Design review of the part built by this model. Coordinates are the model's own, in mm. A direction names the side the tool comes from. Give positions to 0.01 mm unless a question says otherwise; leave off trailing zeros. Write each loop counter-clockwise with the first axis right and the second up, starting at its lowest first coordinate (ties: lowest second). Pieces come first, ordered by that corner, then holes.
```python
from build123d import *

# Parameters (mm, degrees)
SCHIZZO1_R                   = 15
ESTRUSIONE_ESTRUSIONE1_DEPTH = 3.781092502
SCHIZZO2_R                   = 1.625
SCHIZZO2_R_2                 = 1.3
TAGLIO_ESTRUSIONE1_DEPTH     = 4.781092502
SCHIZZO3_R                   = 1.3
TAGLIO_ESTRUSIONE2_DEPTH     = 1.6


with BuildPart() as part:
    # Schizzo1 → Estrusione-Estrusione1 (new body)
    with BuildSketch(Plane.XY):
        Circle(SCHIZZO1_R)
    extrude(amount=ESTRUSIONE_ESTRUSIONE1_DEPTH)

    # Schizzo2 → Taglio-Estrusione1 (cut, through all)
    with BuildSketch(Plane.XY.offset(3.781092502)):
        with Locations((12, 0)):
            Circle(SCHIZZO2_R)
        with Locations((-6, 10.392304845)):
            Circle(SCHIZZO2_R)
        with Locations((-6, -10.392304845)):
            Circle(SCHIZZO2_R)
        Circle(SCHIZZO2_R_2)
    extrude(amount=-TAGLIO_ESTRUSIONE1_DEPTH, mode=Mode.SUBTRACT)

    # Schizzo3 → Taglio-Estrusione2 (cut)
    with BuildSketch(Plane.XY.offset(3.781092502)):
        with BuildLine():
            Line((2.324693054, 3.969357908), (-7.234922947, -1.579015265))
            ThreePointArc((-7.234922947, -1.579015265), (-8.052751546, -4.652222254), (-4.980479907, -5.473557626))
            Line((-4.980479907, -5.473557626), (7.230479097, 1.576442841))
            ThreePointArc((7.230479097, 1.576442841), (8.058653282, 4.641964906), (4.996568233, 5.482758079))
            Line((4.996568233, 5.482758079), (2.324693054, 3.969357908))
        make_face()
        Circle(SCHIZZO3_R, mode=Mode.SUBTRACT)
        with BuildLine():
            Line((-4.599733028, -0.049558742), (-1.133047311, 1.962495511))
            Line((-1.133047311, 1.962495511), (-2.3, 3.983716857))
            ThreePointArc((-2.3, 3.983716857), (-3.996048921, 2.278506752), (-4.599733028, -0.049558742))
        make_face()
        with BuildLine():
            Line((-2.3, 3.983716857), (-1.133047311, 1.962495511))
            Line((-1.133047311, 1.962495511), (2.324693054, 3.969357908))
            ThreePointArc((2.324693054, 3.969357908), (0.014282212, 4.599977828), (-2.3, 3.983716857))
        make_face()
        with BuildLine():
            ThreePointArc((-2.349640269, -3.954641653), (2.3, -3.983716857), (4.599640269, 0.057527336))
            Line((4.599640269, 0.057527336), (-2.349640269, -3.954641653))
        make_face()
    extrude(amount=-TAGLIO_ESTRUSIONE2_DEPTH, mode=Mode.SUBTRACT)


solid = part.part
```
(1) Mouldability with a two-part tool opening along Y and no side actions: class faces 3 (the face through (3, 0, 0)), 4 (the face through (-14.985, 0.66, 1.864)), 5 (the face through (-0.17, 1.29, 1.11)), 6 (the face through (10.377, 0.071, 1.917)) as pulls with the +Y half, pulls with the -Y half, needs draft (parallel to the pull), parting line crosses it, or undercut.
Resolved:
face 3: needs draft
face 4: parting line crosses it
face 5: undercut
face 6: undercut
(2) Clearance check with flat-ended pins moving along their axes: P1, Ø1.6, axis at x = 0, y = 0, coming from the -Z side; P2, Ø1, axis at y = -4, z = 0.5, coming from the +X side; P3, Ø1, axis at x = 6, z = 2, coming from the -Y side; P4, Ø2, axis at x = 4.5, z = 2.5, coming from the +Y side. State where each tip first meets the part, or that it passes through.
Resolved:
P1: passes through
P2: stops at x = 14.59
P3: stops at y = -13.96
P4: stops at y = 14.59
(3) Consider section D-D, the plane z = 2.9. Give the boundary of the cut face in (x, y) (3 decimals), then the cut area to 3 significant figures.
Resolved:
outline: circle Ø30 at (0, 0); hole circle Ø3.25 at (-6, -10.392); hole circle Ø3.25 at (-6, 10.392); hole (-7.235, -1.579) arc R2.25 ccw to (-4.98, -5.474) - (-2.35, -3.955) arc R4.6 ccw to (4.6, 0.058) - (7.23, 1.576) arc R2.25 ccw to (4.997, 5.483) - (2.325, 3.969) arc R4.6 ccw to (-4.6, -0.05) - close; hole circle Ø3.25 at (12, 0)
area: 576 mm2
(4) Consider section B-B, the plane x = -6. Give the boundary of the cut face in (y, z), then the cut area to 3 significant figures.
Resolved:
outline: (-13.75, 0) - (-12.02, 0) - (-12.02, 3.78) - (-13.75, 3.78) - close; (-8.77, 0) - (8.77, 0) - (8.77, 3.78) - (-0.86, 3.78) - (-0.86, 2.18) - (-5.77, 2.18) - (-5.77, 3.78) - (-8.77, 3.78) - close; (12.02, 0) - (13.75, 0) - (13.75, 3.78) - (12.02, 3.78) - close
area: 71.5 mm2
(5) Consider section C-C, the plane y = 0.75. Give the boundary of the cut face in (x, z).
Resolved:
outline: (-14.98, 0) - (-1.06, 0) - (-1.06, 2.18) - (-4.54, 2.18) - (-4.54, 3.78) - (-14.98, 3.78) - close; (1.06, 0) - (10.56, 0) - (10.56, 3.78) - (5.8, 3.78) - (5.8, 2.18) - (1.06, 2.18) - close; (13.44, 0) - (14.98, 0) - (14.98, 3.78) - (13.44, 3.78) - close
(6) To check wall thickness, follow L1, parallel to Y at x = 0, z = 1.6; L2, parallel to Y at x = -6, z = 2.9; L3, parallel to Y at x = -6, z = 2.05. State the ranges of each line that lie inside material, in increasing order.
Resolved:
L1: y = -15 to -1.3, 1.3 to 15
L2: y = -13.75 to -12.02, -8.77 to -5.77, -0.86 to 8.77, 12.02 to 13.75
L3: y = -13.75 to -12.02, -8.77 to 8.77, 12.02 to 13.75
(7) Consider section A-A, the plane x = 0. Give the boundary of the cut face in (y, z).
Resolved:
outline: (-15, 0) - (-1.3, 0) - (-1.3, 2.18) - (-4.6, 2.18) - (-4.6, 3.78) - (-15, 3.78) - close; (1.3, 0) - (15, 0) - (15, 3.78) - (4.6, 3.78) - (4.6, 2.18) - (1.3, 2.18) - close
(8) Tool access review of faces 1 (the face through (5.9, 0.81, 2.99)), 2 (the face through (-7.29, -11.38, 1.92)): name each direction out of +Z, -Z, +X, -X, +Y, -Y from which nothing blocks a thin tool from reaching the whole face with its end or side.
Resolved:
face 1: +Z
face 2: +Z, -Z
